Here's how the part is built. I have some questions about the finished solid (model axes, mm). Face numbers are marked on the shaded views. A direction names the side the tool comes from. Give positions to 0.01 mm unless a question says otherwise; leave off trailing zeros. Write each loop counter-clockwise with the first axis right and the second up, starting at its lowest first coordinate (ties: lowest second). Pieces come first, ordered by that corner, then holes. Notation, with made-up numbers: (55.25, -15) -> (96.25, -15) arc R18 ccw to (96.25, 10) -> close; hole circle Ø7 at (-36, -23). An arc over 180 degrees is marked (long way). Return JSON: item names as keys, results as strings.
from build123d import *

# Parameters (mm, degrees)
BOSS_EXTRUDE1_DEPTH = 50


with BuildPart() as part:
    # Sketch2 → Boss-Extrude1 (new body)
    with BuildSketch(Plane.XY):
        with BuildLine():
            Line((-32.5, 0), (-32.5, -32.5))
            Line((-32.5, -32.5), (-56.553245639, -32.5))
            Line((-56.553245639, -32.5), (-56.553245639, -22.5))
            Line((-56.553245639, -22.5), (-40.8373789, -22.5))
            Line((-40.8373789, -22.5), (-40.8373789, -2.010804855))
            ThreePointArc((-40.8373789, -2.010804855), (-20.267475074, 35.510059219), (22.5, 34.139198169))
            Line((22.5, 34.139198169), (22.5, 54.513252466))
            Line((22.5, 54.513252466), (32.5, 54.513252466))
            Line((32.5, 54.513252466), (32.5, 16.381694729))
            Line((32.5, 16.381694729), (28.069379719, 16.381694729))
            ThreePointArc((28.069379719, 16.381694729), (-8.485138748, 31.372797459), (-32.5, 0))
        make_face()
    extrude(amount=-BOSS_EXTRUDE1_DEPTH)


solid = part.part
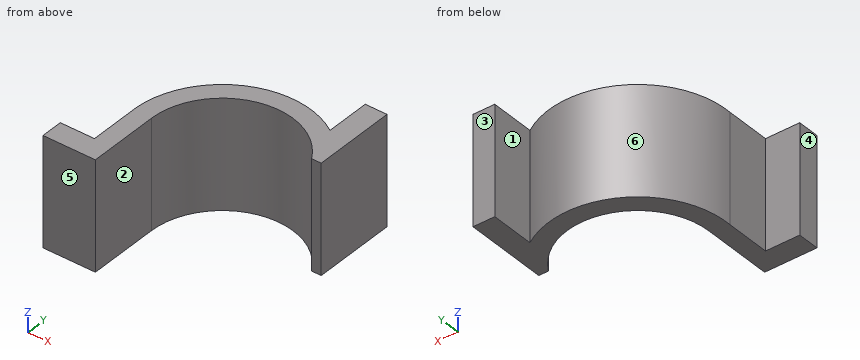
1. Which directions (+Z, -Z, +X, -X, +Y, -Y) give clear straight access to the entire face, cutting with the end or side of a thin tool? Please do the marked faces 1, 2 and 3.
Taken from the geometry:
{"face 1": "+Z, -Z, +Y", "face 2": "+Z, -Z, +X, -Y", "face 3": "+Z, -Z, +X, -X, +Y"}
2. Suppose I cut it at C-C, the plane x = -27. List the corners of the cut face in (y, z) for me.
Taken from the geometry:
{"outline": "(18.09, -50) -> (30.7, -50) -> (30.7, 0) -> (18.09, 0) -> close"}
3. If we mould it in two halves opening along X, with no side actions, what happens to the marked faces 4, 5 and 6? For each: released by +X, released by -X, zero draft, split by the parting line, or undercut.
Taken from the geometry:
{"face 4": "released by -X", "face 5": "zero draft", "face 6": "undercut"}
4. Suppose I cut it at B-B, the plane y = 45. List the corners of the cut face in (x, z) for me, and give its area (3 significant figures).
Taken from the geometry:
{"outline": "(22.5, -50) -> (32.5, -50) -> (32.5, 0) -> (22.5, 0) -> close", "area": "500 mm²"}
5. For pin 1 Ø17.5 at (x, z) = (-51.5, -25) entering from +Y; pin 2 Ø12 at (y, z) = (11, -39.5) entering from -X; pin 3 Ø4 at (x, z) = (-39.5, -28.5) entering from +Y; pin 4 Ø4 at (x, y) = (-43, -21.5) entering from -Z, each with a flat end and sliding along its axis, tell me the tip position at first contact or that it passes through.
Taken from the geometry:
{"pin 1": "stops at y = -22.5", "pin 2": "stops at x = -40.58", "pin 3": "stops at y = 16.29", "pin 4": "stops at z = -50"}
6. Suppose I cut it at A-A, the plane z = -21. List the corners of the cut face in (x, y) for me.
Taken from the geometry:
{"outline": "(-56.55, -32.5) -> (-32.5, -32.5) -> (-32.5, 0) arc R32.5 cw to (28.07, 16.38) -> (32.5, 16.38) -> (32.5, 54.51) -> (22.5, 54.51) -> (22.5, 34.14) arc R40.89 ccw to (-40.84, -2.01) -> (-40.84, -22.5) -> (-56.55, -22.5) -> close"}
7. If I drill on line 1 (X direction, y = 43, z = -26.5); line 2 (Y direction, x = -44, z = -17); line 3 (X direction, y = -17, z = -44), over which ranges is the centre line in solid material (lowest first)? Write a range as [from, to].
Taken from the geometry:
{"line 1": "x = [22.5, 32.5]", "line 2": "y = [-32.5, -22.5]", "line 3": "x = [-40.84, -32.5]"}
